Verification items for the finished model (mm, model axes). Round coordinates to 2 decimals unless told otherwise and drop trailing zeros. Order: outer loops, then holes, each group sorted by start corner. A loop starts at its lowest first (then second) coordinate and runs counter-clockwise, first axis right, second up. Notation, with made-up numbers: (17.5, -29.75) -> (42.5, -29.75) arc R13 ccw to (42.5, -23.75) -> close; hole circle Ø5 at (-31, 16.5). An arc over 180 degrees is marked (long way). Answer in a Markdown table with one row per item. Add a question column.
```python
from build123d import *

# Parameters (mm, degrees)
SKETCH_1_W          = 60
SKETCH_1_H          = 124.895763786
SKETCH_1_R          = 2
SKETCH_1_R_2        = 3
EXTRUDE_1_DEPTH     = 3
FILLET_2_R          = 5
FILLET_3_R          = 5
FILLET_4_R          = 5
FILLET_5_R          = 5
SKETCH_2_R          = 3
CUT_EXTRUDE_1_DEPTH = 3


with BuildPart() as part:
    # Эскиз1 → Бобышка-Вытянуть1 (new body)
    with BuildSketch(Plane.XY):
        Rectangle(SKETCH_1_W, SKETCH_1_H)
        with Locations((-25, -57.647881893)):
            Circle(SKETCH_1_R, mode=Mode.SUBTRACT)
        with Locations((-25, -31.647881893)):
            Circle(SKETCH_1_R, mode=Mode.SUBTRACT)
        with Locations((-25, 35.532118107)):
            Circle(SKETCH_1_R, mode=Mode.SUBTRACT)
        with Locations((0, -31.647881893)):
            Circle(SKETCH_1_R_2, mode=Mode.SUBTRACT)
        with Locations((0, 35.532118107)):
            Circle(SKETCH_1_R_2, mode=Mode.SUBTRACT)
        with Locations(Location((25, 35.532118107, 0), (0, 0, 180))):
            Circle(SKETCH_1_R, mode=Mode.SUBTRACT)
        with Locations(Location((25, -31.647881893, 0), (0, 0, 180))):
            Circle(SKETCH_1_R, mode=Mode.SUBTRACT)
        with Locations(Location((25, -57.647881893, 0), (0, 0, 180))):
            Circle(SKETCH_1_R, mode=Mode.SUBTRACT)
    extrude(amount=EXTRUDE_1_DEPTH)

    # Скругление2
    fillet_2_edges = [part.edges().sort_by_distance(p)[0] for p in [
        (-30, 62.447881893, 1.5),
    ]]
    fillet(fillet_2_edges, radius=FILLET_2_R)

    # Скругление3
    fillet_3_edges = [part.edges().sort_by_distance(p)[0] for p in [
        (30, 62.447881893, 1.5),
    ]]
    fillet(fillet_3_edges, radius=FILLET_3_R)

    # Скругление4
    fillet_4_edges = [part.edges().sort_by_distance(p)[0] for p in [
        (30, -62.447881893, 1.5),
    ]]
    fillet(fillet_4_edges, radius=FILLET_4_R)

    # Скругление5
    fillet_5_edges = [part.edges().sort_by_distance(p)[0] for p in [
        (-30, -62.447881893, 1.5),
    ]]
    fillet(fillet_5_edges, radius=FILLET_5_R)

    # Эскиз2 → Вырез-Вытянуть1 (cut)
    with BuildSketch(Plane.XY.offset(3)):
        Circle(SKETCH_2_R)
    extrude(amount=-CUT_EXTRUDE_1_DEPTH, mode=Mode.SUBTRACT)


solid = part.part
```
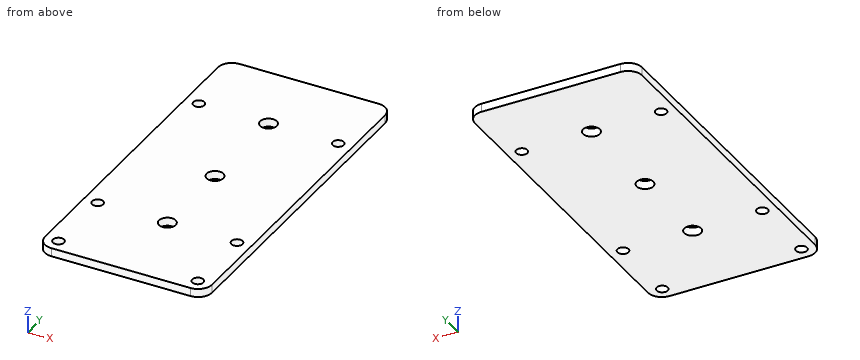
1) Cross-section at B-B, the plane y = 0. Record the boundary of the cut face in (x, z).
2) Thickness scan on L1, parallel to Y at x = 0, z = 1.3; L2, parallel to Y at x = 25, z = 2.1; L3, parallel to X at y = -30, z = 2.35. Record the ranges inside material, lowest first. Write a range as [from, to].
3) Depth check by flat-ended pin: P1, Ø3.5, axis at x = 0, y = 35.53, coming from the +Z side. Enter the tip coordinate at first touch or a pass-through.
4) Cross-section at A-A, the plane x = 0. Record the boundary of the cut face in (y, z), and give its area (3 significant figures).
5) Cross-section at C-C, the plane z = 1.55. Give the number of separate pieces and of enclosed holes in the cut face, and give its area (3 significant figures).
Results below:
| question | item | result |
|---|---|---|
| 1 | outline | (-30, 0) -> (-3, 0) -> (-3, 3) -> (-30, 3) -> close; (3, 0) -> (30, 0) -> (30, 3) -> (3, 3) -> close |
| 2 | L1 | [-62.45, -34.65], [-28.65, -3], [3, 32.53], [38.53, 62.45] |
| 2 | L2 | [-62.45, -59.65], [-55.65, -33.65], [-29.65, 33.53], [37.53, 62.45] |
| 2 | L3 | [-30, -26.13], [-23.87, -2.51], [2.51, 23.87], [26.13, 30] |
| 3 | P1 | through |
| 4 | outline | (-62.45, 0) -> (-34.65, 0) -> (-34.65, 3) -> (-62.45, 3) -> close; (-28.65, 0) -> (-3, 0) -> (-3, 3) -> (-28.65, 3) -> close; (3, 0) -> (32.53, 0) -> (32.53, 3) -> (3, 3) -> close; (38.53, 0) -> (62.45, 0) -> (62.45, 3) -> (38.53, 3) -> close |
| 4 | area | 321 mm² |
| 5 | separate pieces | 1 |
| 5 | enclosed holes | 9 |
| 5 | area | 7,310 mm² |
